Job drawing, mm, ordinate dimensions from the low corner. One solid piece. A direction names the side the tool comes from. Give positions to 0.01 mm unless a question says otherwise; leave off trailing zeros. Loops run counter-clockwise (first coordinate to the right, second up) from the corner with the lowest first, then second, coordinate; pieces in that order, holes last. Notation, with made-up numbers: M 20.25,-36.75 L 77.25,-36.75 A31 cw 77.25,-6.75 Z; hole C 88.25,23 d2. An arc over 180 degrees is marked long. Put each result on its own line as item: value.
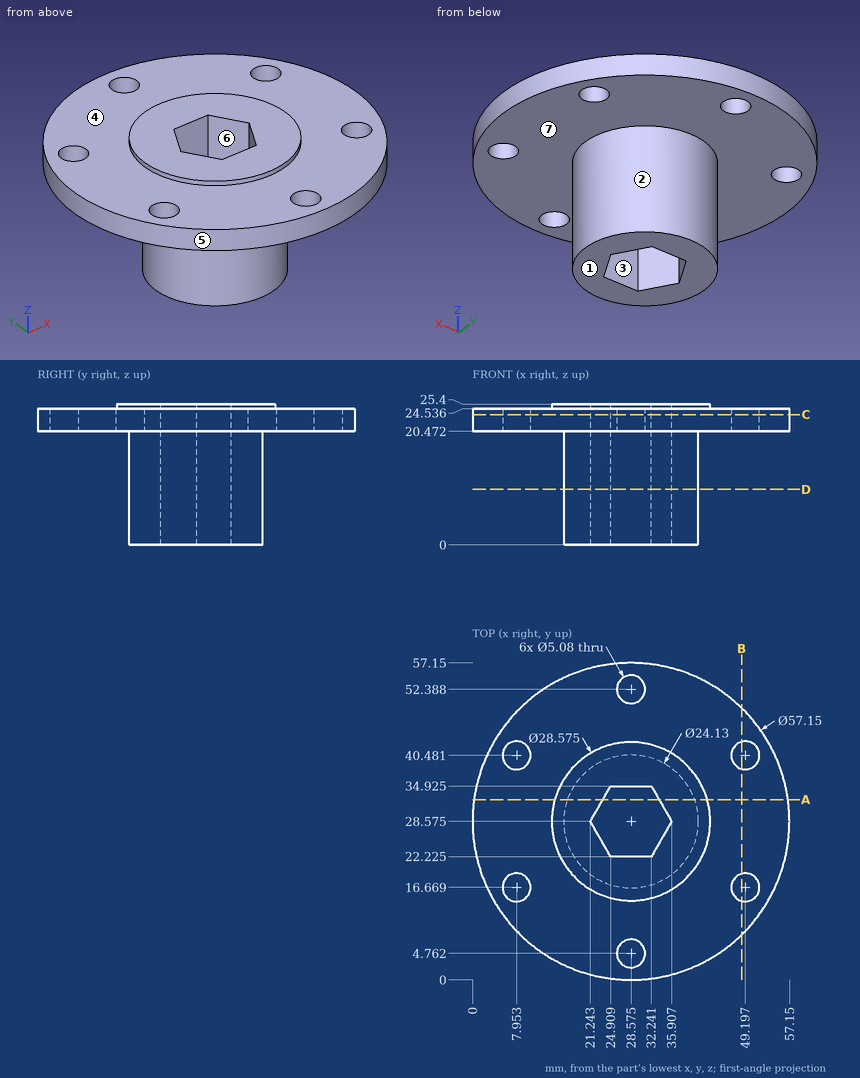
Q1. Drop flat-ended pins along their axis: pin 1 Ø2 at (x, z) = (29.5, 15.5) entering from -Y; pin 2 Ø10 at (x, z) = (16.5, 18) entering from +Y (1 decimal); pin 3 Ø6.5 at (x, y) = (7.95, 40.48) entering from +Z. Give the stop position or say it passes through.
Here are the results:
pin 1: y = 16.51
pin 2: y = 56.1
pin 3: z = 24.54
Q2. Tool access for the marked faces 1, 2, 3 and 4: list every direction of +Z, -Z, +X, -X, +Y, -Y with a clear straight run to the whole face (end or side of a thin tool).
Here are the results:
face 1: -Z, +X, -X, +Y, -Y
face 2: -Z
face 3: +Z, -Z
face 4: +Z
Q3. Probe line 1 (Y direction, x = 51, z = 24) (1 decimal); line 2 (Y direction, x = 6, z = 22.25) (1 decimal); line 3 (Z direction, x = 39, y = 48). List the from-to ranges inside material, lowest first. Write a range as from..to.
Here are the results:
line 1: 10.9..14.9, 18.5..38.7, 42.3..46.3
line 2: 11.1..15, 18.3..38.9, 42.1..46.1
line 3: 20.47..24.54
Q4. Slice it at B-B (x = 48.5). List the corners of the cut face in (y, z), and give its area (3 significant figures).
Here are the results:
outline: M 8.09,20.47 L 14.23,20.47 L 14.23,24.54 L 8.09,24.54 Z; M 19.11,20.47 L 38.04,20.47 L 38.04,24.54 L 19.11,24.54 Z; M 42.92,20.47 L 49.06,20.47 L 49.06,24.54 L 42.92,24.54 Z
area: 127 mm²
Q5. Mould opens along Y. For the marked faces 5, 6 and 7 say: pulls with the +Y half, pulls with the -Y half, needs draft (parallel to the pull), parting line crosses it, or undercut.
Here are the results:
face 5: parting line crosses it
face 6: undercut
face 7: needs draft
Q6. Slice it at C-C (z = 23.5). State how many separate pieces and enclosed holes the cut face has, and give its area (3 significant figures).
Here are the results:
separate pieces: 1
enclosed holes: 7
area: 2,300 mm²
Q7. Slice it at A-A (y = 32.5). List the corners of the cut face in (x, z).
Here are the results:
outline: M 0.27,20.47 L 17.17,20.47 L 17.17,0 L 23.51,0 L 23.51,25.4 L 14.84,25.4 L 14.84,24.54 L 0.27,24.54 Z; M 33.64,0 L 39.98,0 L 39.98,20.47 L 56.88,20.47 L 56.88,24.54 L 42.31,24.54 L 42.31,25.4 L 33.64,25.4 Z
Q8. Slice it at D-D (z = 10). List the corners of the cut face in (x, y) (1 decimal), and give its area (3 significant figures).
Here are the results:
outline: C 28.6,28.6 d24.1; hole M 21.2,28.6 L 24.9,22.2 L 32.2,22.2 L 35.9,28.6 L 32.2,34.9 L 24.9,34.9 Z
area: 318 mm²
